from build123d import *

# Parameters (mm, degrees)
SKETCH1_W           = 6
SKETCH1_H           = 6
BOSS_EXTRUDE1_DEPTH = 5
CUT_EXTRUDE8_DEPTH  = 1
CUT_EXTRUDE11_DEPTH = 12


with BuildPart() as part:
    # Sketch1 → Boss-Extrude1 (new body)
    with BuildSketch(Plane(origin=(0, 0, 0), x_dir=(1, 0, 0), z_dir=(0, 1, 0))):
        Rectangle(SKETCH1_W, SKETCH1_H)
    extrude(amount=BOSS_EXTRUDE1_DEPTH)

    # Sketch9 → Cut-Extrude8 (cut, symmetric)
    with BuildSketch(Plane(origin=(0, 0, 0), x_dir=(0, 0, -1), z_dir=(1, 0, 0))):
        Polygon((3, 5), (-3, 5), (3, 1), align=None)
        Polygon((3, 0), (-3, 2), (-3, 0), align=None)
    extrude(amount=CUT_EXTRUDE8_DEPTH, both=True, mode=Mode.SUBTRACT)

    # Sketch10 → Cut-Extrude11 (cut)
    with BuildSketch(Plane.XY.offset(3)):
        Polygon((-3, 2), (-1, 5), (-3, 5), align=None)
        Polygon((3, 5), (1, 5), (3, 3), align=None)
    extrude(amount=-CUT_EXTRUDE11_DEPTH, mode=Mode.SUBTRACT)


solid = part.part
Build history of the part. All positions in model axes, mm. A direction names the side the tool comes from. Round coordinates to 2 decimals unless told otherwise and drop trailing zeros. Loops run counter-clockwise (first coordinate to the right, second up) from the corner with the lowest first, then second, coordinate; pieces in that order, holes last. Notation, with made-up numbers: (63, 15.5) -> (81, 15.5) arc R6 ccw to (81, 25.5) -> close; hole circle Ø7 at (12, 23). An arc over 180 degrees is marked (long way). One line per item, written item: value. Start each with the question number.
Q1. Drop a flat-ended pin along its axis: pin 1 Ø1 at (x, z) = (2, -2) entering from +Y. Give the stop position or say it passes through.
Q2. 3-axis set-ups, long thin cutter, end or side, ignore diameter. For faces 1 (the face through (0, 0.8, -3)), 2 (the face through (-1, 4, -1)), 3 (the face through (0, 1, 0)): which of +Z, -Z, +X, -X, +Y, -Y reach the whole face in a straight line?
Q3. Cut at D-D on y = 2.6. List the corners of the cut face in (x, z), plus the area to 3 significant figures.
Q4. Cut at B-B on z = -1.5. List the corners of the cut face in (x, y), plus the area to 3 significant figures.
Q5. Cut at A-A on y = 0.4. List the corners of the cut face in (x, z), plus the area to 3 significant figures.
Q6. Cut at C-C on x = 2.5. List the corners of the cut face in (y, z), plus the area to 3 significant figures.
Q7. Probe line 1 along X through (y, z) = (0.6, -0.5); line 2 along X through (y, z) = (4.6, 1); line 3 along Y through (x, z) = (0, -2). List the from-to ranges inside material, lowest first.
Computed:
1. pin 1: y = 4.5
2. face 1: -Z, +X, -X, +Y, -Y
2. face 2: -Z, +Y
2. face 3: +Z, -Y
3. outline: (-2.6, -3) -> (-1, -3) -> (-1, -0.6) -> (1, -0.6) -> (1, -3) -> (3, -3) -> (3, 3) -> (-2.6, 3) -> close
3. area: 28.8 mm²
4. outline: (-3, 0) -> (-1, 0) -> (-1, 0.5) -> (1, 0.5) -> (1, 0) -> (3, 0) -> (3, 3) -> (1, 5) -> (1, 2) -> (-1, 2) -> (-1, 5) -> (-3, 2) -> close
4. area: 18.0 mm²
5. outline: (-3, -3) -> (3, -3) -> (3, 3) -> (1, 3) -> (1, -1.8) -> (-1, -1.8) -> (-1, 3) -> (-3, 3) -> close
5. area: 26.4 mm²
6. outline: (0, -3) -> (3.5, -3) -> (3.5, 3) -> (0, 3) -> close
6. area: 21.0 mm²
7. line 1: -3 to -1, 1 to 3
7. line 2: -1.27 to -1, 1 to 1.4
7. line 3: 0.33 to 1.67
